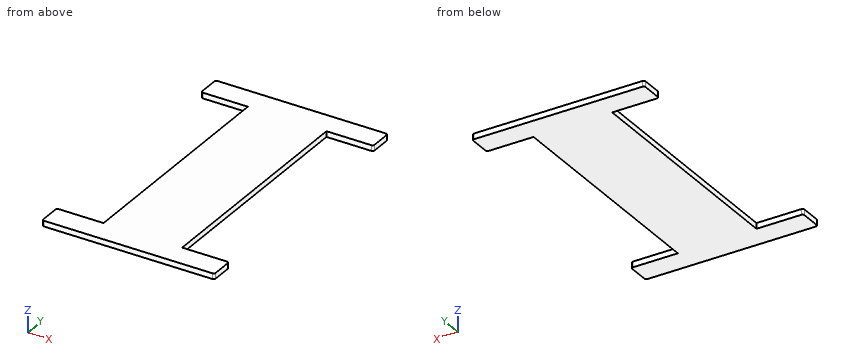
```python
from build123d import *

# Parameters (mm, degrees)
SKETCH_1_W      = 42
SKETCH_1_H      = 149
EXTRUDE_1_DEPTH = 3
SKETCH_2_W      = 25
SKETCH_2_H      = 12.5
EXTRUDE_2_DEPTH = 3
FILLET_1_R      = 1


with BuildPart() as part:
    # 草图1 → 凸台-拉伸1 (new body)
    with BuildSketch(Plane.XY):
        Rectangle(SKETCH_1_W, SKETCH_1_H)
    extrude(amount=EXTRUDE_1_DEPTH)

    # 草图2 → 凸台-拉伸2 (add)
    with BuildSketch(Plane.XY.offset(3)):
        with Locations((33.5, -68.25)):
            Rectangle(SKETCH_2_W, SKETCH_2_H)
        with Locations((-33.5, -68.25)):
            Rectangle(SKETCH_2_W, SKETCH_2_H)
        with Locations((-33.5, 68.25)):
            Rectangle(SKETCH_2_W, SKETCH_2_H)
        with Locations((33.5, 68.25)):
            Rectangle(SKETCH_2_W, SKETCH_2_H)
    extrude(amount=-EXTRUDE_2_DEPTH)

    # 圆角1
    fillet_1_edges = [part.edges().sort_by_distance(p)[0] for p in [
        (46, -74.5, 1.5),
        (46, -62, 1.5),
        (-46, -62, 1.5),
        (-46, -74.5, 1.5),
        (-46, 74.5, 1.5),
        (-46, 62, 1.5),
        (46, 62, 1.5),
        (46, 74.5, 1.5),
    ]]
    fillet(fillet_1_edges, radius=FILLET_1_R)


solid = part.part
```
Model file for the job. Use its own axes, mm. Coordinates: 2 decimals unless noted, no trailing zeros. Write each loop counter-clockwise with the first axis right and the second up, starting at its lowest first coordinate (ties: lowest second). Pieces come first, ordered by that corner, then holes. Notation, with made-up numbers: (-7, 36) - (35, 36) arc R11 ccw to (35, 44) - close; hole circle Ø1 at (45, -8). An arc over 180 degrees is marked (long way). One line per question, with ' | ' between items. Start each with the question number.
Q1. Drill centre lines: line 1 (Y direction, x = 38, z = 2.8); line 2 (X direction, y = -54.5, z = 2.45). Where is each one in solid material? Low to high. Write a range as [from, to].
Q2. Cut at C-C, the plane y = -35. List the corners of the cut face in (x, z).
Q3. Pin check, flat tips, straight feed: pin 1 (0.9 mm diameter, centred on y = -14.5, z = 1.5, fed in from +X); pin 2 (1 mm diameter, centred on x = -6.5, y = -34.5, fed in from -Z). Stop position of each tip, or through.
Q4. Cut at B-B, the plane z = 0.95. List the corners of the cut face in (x, y), then the cut area to 3 significant figures.
Q5. Cut at A-A, the plane x = 38. List the corners of the cut face in (y, z), then the cut area to 3 significant figures.
Answer below:
1) line 1: [-74.5, -62], [62, 74.5] | line 2: [-21, 21]
2) outline: (-21, 0) - (21, 0) - (21, 3) - (-21, 3) - close
3) pin 1: x = 21 | pin 2: z = 0
4) outline: (-46, -73.5) arc R1 ccw to (-45, -74.5) - (45, -74.5) arc R1 ccw to (46, -73.5) - (46, -63) arc R1 ccw to (45, -62) - (21, -62) - (21, 62) - (45, 62) arc R1 ccw to (46, 63) - (46, 73.5) arc R1 ccw to (45, 74.5) - (-45, 74.5) arc R1 ccw to (-46, 73.5) - (-46, 63) arc R1 ccw to (-45, 62) - (-21, 62) - (-21, -62) - (-45, -62) arc R1 ccw to (-46, -63) - close | area: 7,510 mm^2
5) outline: (-74.5, 0) - (-62, 0) - (-62, 3) - (-74.5, 3) - close; (62, 0) - (74.5, 0) - (74.5, 3) - (62, 3) - close | area: 75.0 mm^2
